CAD build for the part. Positions are in the model's coordinates, mm. Face numbers are marked on the shaded views. A direction names the side the tool comes from. Give positions to 0.01 mm unless a question says otherwise; leave off trailing zeros. Loops run counter-clockwise (first coordinate to the right, second up) from the corner with the lowest first, then second, coordinate; pieces in that order, holes last. Notation, with made-up numbers: M 87,37 L 145,37 A19 cw 145,43 Z; hole C 71,45.5 d9. An arc over 180 degrees is marked long. One line per question, with ' | ' between items.
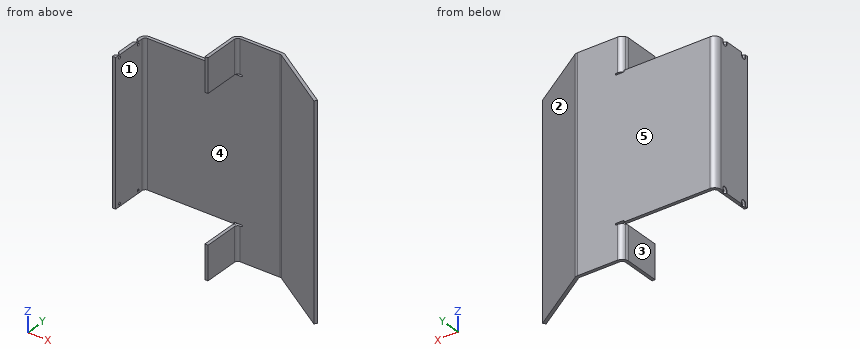
```python
from build123d import *

# Parameters (mm, degrees)
SALIENTE_EXTRUIR1_DEPTH          = 3
BRIDA_DE_ARISTA1_STRIP_W         = 18
BRIDA_DE_ARISTA1_STRIP_H         = 3
BRIDA_DE_ARISTA1_STRIP_CUT_DEPTH = 136
BRIDA_DE_ARISTA1_DEPTH           = 136
CROQUIS5_R                       = 1.25
CORTAR_EXTRUIR1_DEPTH            = 3
CORTAR_EXTRUIR2_DEPTH            = 2
CHAFL_N1_SIZE                    = 1.5
BRIDA_START                      = -100
BRIDA_DE_ARISTA2_DEPTH           = 33.5
BRIDA_START_2                    = 66.5
BRIDA_DE_ARISTA2_2_DEPTH         = 33.5
BRIDA_DE_ARISTA2_3_DEPTH         = 32
BRIDA_START_3                    = 68
BRIDA_DE_ARISTA2_4_DEPTH         = 32
BRIDA_START_4                    = -3
BRIDA_DE_ARISTA2_5_DEPTH         = 7
BRIDA_DE_ARISTA3_STRIP_CUT_DEPTH = 200
BRIDA_DE_ARISTA3_DEPTH           = 200


with BuildPart() as part:
    # Croquis1 → Saliente-Extruir1 (new body)
    with BuildSketch(Plane(origin=(0, 0, 0), x_dir=(1, 0, 0), z_dir=(0, 1, 0))):
        Polygon((-42.5, -68), (42.5, -68), (42.5, -100), (87.5, -100), (87.5, 100), (42.5, 100), (42.5, 68), (-42.5, 68), align=None)
    extrude(amount=SALIENTE_EXTRUIR1_DEPTH)

    # Brida de arista1: sheet metal written as solids
    # Brida de arista1 strip (on a plane across the edge) → Brida de arista1 strip cut (cut)
    with BuildSketch(Plane(origin=(-42.5, 0, 68), x_dir=(1, 0, 0), z_dir=(0, 0, -1))):
        with Locations((-6, -1.5)):
            Rectangle(BRIDA_DE_ARISTA1_STRIP_W, BRIDA_DE_ARISTA1_STRIP_H)
    extrude(amount=BRIDA_DE_ARISTA1_STRIP_CUT_DEPTH, mode=Mode.SUBTRACT)

    # Brida de arista1 section (on a plane across the edge) → Brida de arista1 (add)
    with BuildSketch(Plane(origin=(-42.5, 0, 68), x_dir=(1, 0, 0), z_dir=(0, 0, -1))):
        with BuildLine():
            Line((-3, 3), (-3, 37))
            Line((-3, 37), (0, 37))
            Line((0, 37), (0, 3))
            ThreePointArc((0, 3), (0.878679656, 0.878679656), (3, 0))
            Line((3, 0), (3, -3))
            ThreePointArc((3, -3), (-1.242640687, -1.242640687), (-3, 3))
        make_face()
    extrude(amount=BRIDA_DE_ARISTA1_DEPTH)

    # Croquis5 → Cortar-Extruir1 (cut)
    with BuildSketch(Plane.ZY.offset(45.5)):
        with Locations(Location((65.5, -32, 0), (0, 0, 270))):
            Circle(CROQUIS5_R)
        with Locations(Location((65.5, -8, 0), (0, 0, 270))):
            Circle(CROQUIS5_R)
        with Locations(Location((-65.5, -8, 0), (0, 0, 90))):
            Circle(CROQUIS5_R)
        with Locations(Location((-65.5, -32, 0), (0, 0, 90))):
            Circle(CROQUIS5_R)
    extrude(amount=-CORTAR_EXTRUIR1_DEPTH, mode=Mode.SUBTRACT)

    # Croquis6 → Cortar-Extruir2 (cut)
    with BuildSketch(Plane.ZY.offset(45.5)):
        with BuildLine():
            Line((65.5, -5.5), (68, -5.5))
            Line((68, -5.5), (68, -10.5))
            Line((68, -10.5), (65.5, -10.5))
            ThreePointArc((65.5, -10.5), (63, -8), (65.5, -5.5))
        make_face()
        with BuildLine():
            Line((68, -29.5), (65.5, -29.5))
            ThreePointArc((65.5, -29.5), (63, -32), (65.5, -34.5))
            Line((65.5, -34.5), (68, -34.5))
            Line((68, -34.5), (68, -29.5))
        make_face()
        with BuildLine():
            Line((-65.5, -34.5), (-68, -34.5))
            Line((-68, -34.5), (-68, -29.5))
            Line((-68, -29.5), (-65.5, -29.5))
            ThreePointArc((-65.5, -29.5), (-63, -32), (-65.5, -34.5))
        make_face()
        with BuildLine():
            Line((-68, -10.5), (-65.5, -10.5))
            ThreePointArc((-65.5, -10.5), (-63, -8), (-65.5, -5.5))
            Line((-65.5, -5.5), (-68, -5.5))
            Line((-68, -5.5), (-68, -10.5))
        make_face()
    extrude(amount=-CORTAR_EXTRUIR2_DEPTH, mode=Mode.SUBTRACT)

    # Chaflán1
    # the kernel refuses this chamfer: 1.5 mm, written as the material it adds along each edge
    with BuildSketch(Plane(origin=(-43.5, -5.5, 65.5), x_dir=(-1, 0, 0), z_dir=(0, 0, 1))) as chafl_n1_piece_1_section:
        Polygon((CHAFL_N1_SIZE, 0), (0, CHAFL_N1_SIZE), (0, 0), align=None)
    chafl_n1_piece_1 = extrude(amount=2.5, mode=Mode.PRIVATE)
    chafl_n1_piece_1 = chafl_n1_piece_1 - Plane(origin=(-43.5, -8, 65.5), x_dir=(0, -1, 0), z_dir=(-1, 0, 0)) * Cylinder(1.25, 12, mode=Mode.PRIVATE)
    add(chafl_n1_piece_1)
    with BuildSketch(Plane(origin=(-43.5, -10.5, 68), x_dir=(0, 1, 0), z_dir=(0, 0, -1))) as chafl_n1_piece_2_section:
        Polygon((CHAFL_N1_SIZE, 0), (0, -CHAFL_N1_SIZE), (0, 0), align=None)
    chafl_n1_piece_2 = extrude(amount=2.5, mode=Mode.PRIVATE)
    chafl_n1_piece_2 = chafl_n1_piece_2 - Plane(origin=(-43.5, -8, 65.5), x_dir=(0, -1, 0), z_dir=(-1, 0, 0)) * Cylinder(1.25, 12, mode=Mode.PRIVATE)
    add(chafl_n1_piece_2)
    with BuildSketch(Plane(origin=(-43.5, -29.5, 68), x_dir=(-1, 0, 0), z_dir=(0, 0, -1))) as chafl_n1_piece_3_section:
        Polygon((CHAFL_N1_SIZE, 0), (0, -CHAFL_N1_SIZE), (0, 0), align=None)
    chafl_n1_piece_3 = extrude(amount=2.5, mode=Mode.PRIVATE)
    chafl_n1_piece_3 = chafl_n1_piece_3 - Plane(origin=(-43.5, -32, 65.5), x_dir=(0, -1, 0), z_dir=(-1, 0, 0)) * Cylinder(1.25, 12, mode=Mode.PRIVATE)
    add(chafl_n1_piece_3)
    with BuildSketch(Plane(origin=(-43.5, -34.5, 65.5), x_dir=(0, 1, 0), z_dir=(0, 0, 1))) as chafl_n1_piece_4_section:
        Polygon((CHAFL_N1_SIZE, 0), (0, CHAFL_N1_SIZE), (0, 0), align=None)
    chafl_n1_piece_4 = extrude(amount=2.5, mode=Mode.PRIVATE)
    chafl_n1_piece_4 = chafl_n1_piece_4 - Plane(origin=(-43.5, -32, 65.5), x_dir=(0, -1, 0), z_dir=(-1, 0, 0)) * Cylinder(1.25, 12, mode=Mode.PRIVATE)
    add(chafl_n1_piece_4)
    with BuildSketch(Plane(origin=(-43.5, -34.5, -65.5), x_dir=(-1, 0, 0), z_dir=(0, 0, -1))) as chafl_n1_piece_5_section:
        Polygon((CHAFL_N1_SIZE, 0), (0, CHAFL_N1_SIZE), (0, 0), align=None)
    chafl_n1_piece_5 = extrude(amount=2.5, mode=Mode.PRIVATE)
    chafl_n1_piece_5 = chafl_n1_piece_5 - Plane(origin=(-43.5, -32, -65.5), x_dir=(0, 1, 0), z_dir=(-1, 0, 0)) * Cylinder(1.25, 12, mode=Mode.PRIVATE)
    add(chafl_n1_piece_5)
    with BuildSketch(Plane(origin=(-43.5, -29.5, -68), x_dir=(-1, 0, 0), z_dir=(0, 0, 1))) as chafl_n1_piece_6_section:
        Polygon((CHAFL_N1_SIZE, 0), (0, CHAFL_N1_SIZE), (0, 0), align=None)
    chafl_n1_piece_6 = extrude(amount=2.5, mode=Mode.PRIVATE)
    chafl_n1_piece_6 = chafl_n1_piece_6 - Plane(origin=(-43.5, -32, -65.5), x_dir=(0, 1, 0), z_dir=(-1, 0, 0)) * Cylinder(1.25, 12, mode=Mode.PRIVATE)
    add(chafl_n1_piece_6)
    with BuildSketch(Plane(origin=(-43.5, -10.5, -68), x_dir=(-1, 0, 0), z_dir=(0, 0, 1))) as chafl_n1_piece_7_section:
        Polygon((CHAFL_N1_SIZE, 0), (0, -CHAFL_N1_SIZE), (0, 0), align=None)
    chafl_n1_piece_7 = extrude(amount=2.5, mode=Mode.PRIVATE)
    chafl_n1_piece_7 = chafl_n1_piece_7 - Plane(origin=(-43.5, -8, -65.5), x_dir=(0, 1, 0), z_dir=(-1, 0, 0)) * Cylinder(1.25, 12, mode=Mode.PRIVATE)
    add(chafl_n1_piece_7)
    with BuildSketch(Plane(origin=(-43.5, -5.5, -65.5), x_dir=(-1, 0, 0), z_dir=(0, 0, -1))) as chafl_n1_piece_8_section:
        Polygon((CHAFL_N1_SIZE, 0), (0, -CHAFL_N1_SIZE), (0, 0), align=None)
    chafl_n1_piece_8 = extrude(amount=2.5, mode=Mode.PRIVATE)
    chafl_n1_piece_8 = chafl_n1_piece_8 - Plane(origin=(-43.5, -8, -65.5), x_dir=(0, 1, 0), z_dir=(-1, 0, 0)) * Cylinder(1.25, 12, mode=Mode.PRIVATE)
    add(chafl_n1_piece_8)
    with BuildSketch(Plane(origin=(-43.5, -8, -65.5), x_dir=(0, -1, 0), z_dir=(0, 0, -1))) as chafl_n1_piece_9_section:
        Polygon((2.5, CHAFL_N1_SIZE), (2.5 - CHAFL_N1_SIZE, 0), (2.5, 0), align=None)
    chafl_n1_piece_9 = revolve(axis=Axis((-43.5, -8, -65.5), (-1, 0, 0)), revolution_arc=180, mode=Mode.PRIVATE)
    chafl_n1_piece_9 = chafl_n1_piece_9 - Plane(origin=(-43.5, -8, -65.5), x_dir=(0, 1, 0), z_dir=(-1, 0, 0)) * Cylinder(1.25, 11, mode=Mode.PRIVATE)
    add(chafl_n1_piece_9)
    with BuildSketch(Plane(origin=(-43.5, -32, -65.5), x_dir=(0, 1, 0), z_dir=(0, 0, -1))) as chafl_n1_piece_10_section:
        Polygon((2.5, -CHAFL_N1_SIZE), (2.5 - CHAFL_N1_SIZE, 0), (2.5, 0), align=None)
    chafl_n1_piece_10 = revolve(axis=Axis((-43.5, -32, -65.5), (1, 0, 0)), revolution_arc=180, mode=Mode.PRIVATE)
    chafl_n1_piece_10 = chafl_n1_piece_10 - Plane(origin=(-43.5, -32, -65.5), x_dir=(0, 1, 0), z_dir=(-1, 0, 0)) * Cylinder(1.25, 11, mode=Mode.PRIVATE)
    add(chafl_n1_piece_10)
    with BuildSketch(Plane(origin=(-43.5, -32, 65.5), x_dir=(0, 1, 0), z_dir=(0, 0, 1))) as chafl_n1_piece_11_section:
        Polygon((2.5 - CHAFL_N1_SIZE, 0), (2.5, CHAFL_N1_SIZE), (2.5, 0), align=None)
    chafl_n1_piece_11 = revolve(axis=Axis((-43.5, -32, 65.5), (-1, 0, 0)), revolution_arc=180, mode=Mode.PRIVATE)
    chafl_n1_piece_11 = chafl_n1_piece_11 - Plane(origin=(-43.5, -32, 65.5), x_dir=(0, -1, 0), z_dir=(-1, 0, 0)) * Cylinder(1.25, 11, mode=Mode.PRIVATE)
    add(chafl_n1_piece_11)
    with BuildSketch(Plane(origin=(-43.5, -8, 65.5), x_dir=(0, -1, 0), z_dir=(0, 0, 1))) as chafl_n1_piece_12_section:
        Polygon((2.5 - CHAFL_N1_SIZE, 0), (2.5, -CHAFL_N1_SIZE), (2.5, 0), align=None)
    chafl_n1_piece_12 = revolve(axis=Axis((-43.5, -8, 65.5), (1, 0, 0)), revolution_arc=180, mode=Mode.PRIVATE)
    chafl_n1_piece_12 = chafl_n1_piece_12 - Plane(origin=(-43.5, -8, 65.5), x_dir=(0, -1, 0), z_dir=(-1, 0, 0)) * Cylinder(1.25, 11, mode=Mode.PRIVATE)
    add(chafl_n1_piece_12)

    # Brida de arista2: read off the stored shape, not the designer's step
    # Brida de arista2 outline → Brida de arista2 (cut)
    with BuildSketch(Plane.XY.offset(BRIDA_START)):
        with BuildLine():
            Line((42.5, 0), (43.303847577, 0))
            ThreePointArc((43.303847577, 0), (45.5, 2.196152423), (48.5, 3))
            Line((48.5, 3), (42.5, 3))
            Line((42.5, 3), (42.5, 0))
        make_face()
    extrude(amount=BRIDA_DE_ARISTA2_DEPTH, mode=Mode.SUBTRACT)

    # Brida de arista2 2 outline → Brida de arista2 2 (cut)
    with BuildSketch(Plane.XY.offset(BRIDA_START_2)):
        with BuildLine():
            Line((42.5, 0), (43.303847577, 0))
            ThreePointArc((43.303847577, 0), (45.5, 2.196152423), (48.5, 3))
            Line((48.5, 3), (42.5, 3))
            Line((42.5, 3), (42.5, 0))
        make_face()
    extrude(amount=BRIDA_DE_ARISTA2_2_DEPTH, mode=Mode.SUBTRACT)

    # Brida de arista2 3 outline → Brida de arista2 3 (add)
    with BuildSketch(Plane.XY.offset(BRIDA_START)):
        with BuildLine():
            Line((42.5, -37), (45.5, -37))
            Line((45.5, -37), (45.5, -3))
            ThreePointArc((45.5, -3), (46.378679656, -0.878679656), (48.5, 0))
            Line((48.5, 0), (43.303847577, 0))
            ThreePointArc((43.303847577, 0), (42.704445042, -1.447085729), (42.5, -3))
            Line((42.5, -3), (42.5, -37))
        make_face()
    extrude(amount=BRIDA_DE_ARISTA2_3_DEPTH)

    # Brida de arista2 4 outline → Brida de arista2 4 (add)
    with BuildSketch(Plane.XY.offset(BRIDA_START_3)):
        with BuildLine():
            Line((42.5, -37), (45.5, -37))
            Line((45.5, -37), (45.5, -3))
            ThreePointArc((45.5, -3), (46.378679656, -0.878679656), (48.5, 0))
            Line((48.5, 0), (43.303847577, 0))
            ThreePointArc((43.303847577, 0), (42.704445042, -1.447085729), (42.5, -3))
            Line((42.5, -3), (42.5, -37))
        make_face()
    extrude(amount=BRIDA_DE_ARISTA2_4_DEPTH)

    # Brida de arista2 5 outline → Brida de arista2 5 (cut)
    with BuildSketch(Plane(origin=(0, 0, 0), x_dir=(1, 0, 0), z_dir=(0, 1, 0)).offset(BRIDA_START_4)):
        with BuildLine():
            Line((50, -66.5), (43, -66.5))
            Line((43, -66.5), (43, -68))
            Line((43, -68), (50, -68))
            ThreePointArc((50, -68), (50.75, -67.25), (50, -66.5))
        make_face()
        with BuildLine():
            Line((43, 68), (43, 66.5))
            Line((43, 66.5), (50, 66.5))
            ThreePointArc((50, 66.5), (50.75, 67.25), (50, 68))
            Line((50, 68), (43, 68))
        make_face()
    extrude(amount=BRIDA_DE_ARISTA2_5_DEPTH, mode=Mode.SUBTRACT)

    # Brida de arista3: sheet metal written as solids
    # Brida de arista3 strip (on a plane across the edge) → Brida de arista3 strip cut (cut)
    with BuildSketch(Plane(origin=(87.5, 0, -100), x_dir=(-0.5446390350150233, -0.8386705679454266, 0), z_dir=(0, 0, 1))):
        Polygon((-11.835526038, 12.716876498), (-2.032023408, -2.379193725), (0.483988296, -0.74527662), (-9.319514334, 14.350793603), align=None)
    extrude(amount=BRIDA_DE_ARISTA3_STRIP_CUT_DEPTH, mode=Mode.SUBTRACT)

    # Brida de arista3 section (on a plane across the edge) → Brida de arista3 (add)
    with BuildSketch(Plane(origin=(87.5, 0, -100), x_dir=(-0.5446390350150233, -0.8386705679454266, 0), z_dir=(0, 0, 1))):
        with BuildLine():
            Line((-3, 0.888640485), (-3, 72.111359515))
            Line((-3, 72.111359515), (0, 72.111359515))
            Line((0, 72.111359515), (0, 0.888640485))
            ThreePointArc((0, 0.888640485), (0.123540795, 0.036594451), (0.483988296, -0.74527662))
            Line((0.483988296, -0.74527662), (-2.032023408, -2.379193725))
            ThreePointArc((-2.032023408, -2.379193725), (-2.752918409, -0.815451583), (-3, 0.888640485))
        make_face()
    extrude(amount=BRIDA_DE_ARISTA3_DEPTH)


solid = part.part
```
Item 1: Drop flat-ended pins along their axis: P1, Ø5, axis at y = -12, z = -34.5, coming from the +X side; P2, Ø12, axis at y = -13.5, z = 31, coming from the +X side; P3, Ø3, axis at y = -32, z = -65.5, coming from the +X side. Give the stop position or say it passes through.
Conclusion:
P1: x = 115.34 | P2: x = 123.04 | P3: x = 144.59
Item 2: Saw through at D-D on x = 93. Give the cut face in (y, z).
Conclusion:
outline: M -3.57,-100 L 0.01,-100 L 0.01,100 L -3.57,100 Z
Item 3: 3-axis set-ups, long thin cutter, end or side, ignore diameter. For the marked faces 1 and 2: which of +Z, -Z, +X, -X, +Y, -Y reach the whole face in a straight line?
Conclusion:
face 1: +Z, -Z, -Y | face 2: +Z, -Z, +X, +Y
Item 4: Mould opens along X. For the marked faces 3, 4 and 5 say: pulls with the +X half, pulls with the -X half, needs draft (parallel to the pull), parting line crosses it, or undercut.
Conclusion:
face 3: pulls with the -X half | face 4: undercut | face 5: needs draft
Item 5: Drill centre lines: line 1 along Z through (x, y) = (-43, -8); line 2 along Y through (x, z) = (-42.8, 65.5); line 3 along Y through (x, z) = (-42.95, -65.5). Where is each one in solid material? Low to high. Write a range as [from, to].
Conclusion:
line 1: [-68, -66.75], [-64.25, 64.25], [66.75, 68] | line 2: [-37, -33.25], [-30.75, -9.25], [-6.75, 2.01] | line 3: [-37, -33.25], [-30.75, -9.25], [-6.75, 1.91]
Item 6: Saw through at B-B on x = 10. Give the cut face in (y, z).
Conclusion:
outline: M 0,-68 L 3,-68 L 3,68 L 0,68 Z
Item 7: Saw through at C-C on z = -82.5. Give the cut face in (x, y).
Conclusion:
outline: M 42.5,-37 L 45.5,-37 L 45.5,-3 A3 cw 48.5,0 L 86.61,0 A3 cw 88.25,-0.48 L 147.98,-39.27 L 149.61,-36.76 L 89.88,2.03 A6 ccw 86.61,3 L 48.5,3 A6 ccw 42.5,-3 Z
Item 8: Saw through at A-A on z = 22. Give the cut face in (x, y).
Conclusion:
outline: M -45.5,-37 L -42.5,-37 L -42.5,-3 A3 cw -39.5,0 L 86.61,0 A3 cw 88.25,-0.48 L 147.98,-39.27 L 149.61,-36.76 L 89.88,2.03 A6 ccw 86.61,3 L -39.5,3 A6 ccw -45.5,-3 Z
